```python
from build123d import *

# Parameters (mm, degrees)
SKETCH2_R           = 2.127
BOSS_EXTRUDE1_DEPTH = 11.0998
SKETCH3_W           = 24.110565092
SKETCH3_H           = 30.85676152
CUT_EXTRUDE1_DEPTH  = 11.0998


with BuildPart() as part:
    # Sketch2 → Boss-Extrude1 (new body)
    with BuildSketch(Plane.XY):
        with BuildLine():
            Line((-5.032244852, -170.140769418), (-3.337033957, -142.465103356))
            ThreePointArc((-3.337033957, -142.465103356), (-4.366318267, -139.620020754), (-7.144640499, -138.422169855))
            Line((-7.144640499, -138.422169855), (-15.698665552, -138.4327981))
            ThreePointArc((-15.698665552, -138.4327981), (-18.474002587, -139.637549336), (-19.496213787, -142.48518089))
            Line((-19.496213787, -142.48518089), (-17.732235049, -170.156548962))
            ThreePointArc((-17.732235049, -170.156548962), (-11.374511927, -176.368472831), (-5.032244852, -170.140769418))
        make_face()
        with Locations((-11.409226923, -148.428494397)):
            Circle(SKETCH2_R, mode=Mode.SUBTRACT)
        with Locations((-11.380823745, -171.288476752)):
            Circle(SKETCH2_R, mode=Mode.SUBTRACT)
    extrude(amount=BOSS_EXTRUDE1_DEPTH)

    # Sketch3 → Cut-Extrude1 (cut)
    with BuildSketch(Plane.XY.offset(11.0998)):
        with Locations((-9.740364604, -166.396875157)):
            Rectangle(SKETCH3_W, SKETCH3_H)
    extrude(amount=-CUT_EXTRUDE1_DEPTH, mode=Mode.SUBTRACT)


solid = part.part
```
Read the model definition and answer for the solid it produces. Units are mm, in the model's axes. Coordinates: 2 decimals unless noted, no trailing zeros. Order: outer loops, then holes, each group sorted by start corner. A loop starts at its lowest first (then second) coordinate and runs counter-clockwise, first axis right, second up. Notation, with made-up numbers: (-3.5, 89) - (8.5, 89) arc R21 cw to (8.5, 93) - close; hole circle Ø4 at (18.25, 80). An arc over 180 degrees is marked (long way). Answer as a JSON object with one key per item and string values. Group by question number.
Item 1: Section D-D (x = -5.75) is taken. Give the vertices of the cut face in (y, z).
Item 2: Consider probe 1 along X at (y, z) = (-147.25, 3.25); probe 2 along Y at (x, z) = (-13.75, 4); probe 3 along Y at (x, z) = (-9.75, 4.75). Determine where each line is inside the solid, lowest interval first. Write a range as from..to.
Item 3: Section B-B (z = 6.5) is taken. Give the vertices of the cut face in (x, y).
Item 4: Section A-A (y = -146.75) is taken. Give the vertices of the cut face in (x, z).
Item 5: Section C-C (x = -13) is taken. Give the vertices of the cut face in (y, z), plus the area to 3 significant figures.
Item 6: The mould has two halves that part along X. Classify faces 1 (the face through (-18.444, -139.606, 5.472)), 2 (the face through (-11.69, -146.32, 5.47)), 3 (the face through (-12, -145, 0)): +X half, -X half, draft (parallel to the pull), parting line (faces both ways), or undercut.
Item 7: Flat-ended cylindrical pins translate along their axes: P1, Ø1.5, axis at x = -14, z = 4, coming from the +Y side; P2, Ø2, axis at y = -141, z = 3, coming from the +X side; P3, Ø3.5, axis at x = -11.41, y = -148.43, coming from the +Z side. Find the tip coordinate at first contact, or state that the pin passes through.
Results are:
{
 "1": {"outline": "(-150.97, 0) - (-138.68, 0) - (-138.68, 11.1) - (-150.97, 11.1) - close"},
 "2": {"probe 1": "x = -19.19..-13.18, -9.64..-3.63", "probe 2": "y = -150.97..-138.43", "probe 3": "y = -150.97..-149.76, -147.1..-138.43"},
 "3": {"outline": "(-19.5, -142.49) - (-18.96, -150.97) - (-3.86, -150.97) - (-3.34, -142.47) arc R3.81 ccw to (-7.14, -138.42) - (-15.7, -138.43) arc R3.81 ccw to start; hole circle Ø4.25 at (-11.41, -148.43)"},
 "4": {"outline": "(-19.22, 0) - (-12.72, 0) - (-12.72, 11.1) - (-19.22, 11.1) - close; (-10.1, 0) - (-3.6, 0) - (-3.6, 11.1) - (-10.1, 11.1) - close"},
 "5": {"outline": "(-150.97, 0) - (-149.84, 0) - (-149.84, 11.1) - (-150.97, 11.1) - close; (-147.02, 0) - (-138.43, 0) - (-138.43, 11.1) - (-147.02, 11.1) - close", "area": "108 mm^2"},
 "6": {"face 1": "-X half", "face 2": "undercut", "face 3": "draft"},
 "7": {"P1": "stops at y = -138.43", "P2": "stops at x = -3.34", "P3": "passes through"}
}
